from build123d import *
from build123d.topology import SkipClean

# Parameters (mm, degrees)
SKETCH_1_R          = 5.5
SKETCH_1_R_2        = 4.1
EXTRUDE_1_DEPTH     = 12.5
SKETCH_3_R          = 5.5
EXTRUDE_2_DEPTH     = 20
SKETCH_4_R          = 4.1
CUT_EXTRUDE_2_DEPTH = 22.5
SKETCH_5_R          = 4.1
CUT_EXTRUDE_3_DEPTH = 45


with BuildPart() as part:
    # 草图1 → 凸台-拉伸1 (new, symmetric)
    with BuildSketch(Plane(origin=(0, 0, 0), x_dir=(0, 0, -1), z_dir=(1, 0, 0))):
        Circle(SKETCH_1_R)
        Circle(SKETCH_1_R_2, mode=Mode.SUBTRACT)
    extrude(amount=EXTRUDE_1_DEPTH, both=True)

    # 草图3 → 凸台-拉伸2 (add)
    with BuildSketch(Plane(origin=(0, 0, 0), x_dir=(1, 0, 0), z_dir=(0, 1, 0))):
        with Locations(Location((0, 0, 0), (0, 0, 270))):
            Circle(SKETCH_3_R)
    extrude(amount=EXTRUDE_2_DEPTH)

    # 草图4 → 切除-拉伸2 (cut, symmetric)
    with SkipClean():  # the faces are left unmerged after this step: merging them gives an invalid solid
        with BuildSketch(Plane(origin=(0, 0, 0), x_dir=(0, 0, -1), z_dir=(1, 0, 0))):
            Circle(SKETCH_4_R)
        extrude(amount=CUT_EXTRUDE_2_DEPTH, both=True, mode=Mode.SUBTRACT)

    # 草图5 → 切除-拉伸3 (cut)
    with BuildSketch(Plane(origin=(0, 0, 0), x_dir=(1, 0, 0), z_dir=(0, 1, 0))):
        with Locations(Location((0, 0, 0), (0, 0, 270))):
            Circle(SKETCH_5_R)
    extrude(amount=CUT_EXTRUDE_3_DEPTH, mode=Mode.SUBTRACT)


solid = part.part
Can you work these out from the model? Positions are in its coordinate system, mm. A direction names the side the tool comes from. Give positions to 0.01 mm unless a question says otherwise; leave off trailing zeros. Order: outer loops, then holes, each group sorted by start corner. A loop starts at its lowest first (then second) coordinate and runs counter-clockwise, first axis right, second up. Notation, with made-up numbers: M 40.5,76 L 66.5,76 A11 cw 66.5,82 Z; hole C 9,35.5 d2. An arc over 180 degrees is marked long. Use one line per item in the form item = value.
Item 1: If we section it at A-A, the plane z = 0: Write out the boundary of the cut face in (x, y).
Values follow:
outline = M -12.5,-5.5 L 12.5,-5.5 L 12.5,-4.1 L -12.5,-4.1 Z; M -12.5,4.1 L -4.1,4.1 L -4.1,20 L -5.5,20 L -5.5,5.5 L -12.5,5.5 Z; M 4.1,4.1 L 12.5,4.1 L 12.5,5.5 L 5.5,5.5 L 5.5,20 L 4.1,20 Z
Item 2: If we section it at B-B, the plane x = 0: Write out the boundary of the cut face in (y, z).
Values follow:
outline = M 0,-5.5 L 20,-5.5 L 20,-4.1 L 0,-4.1 A4.1 cw 0,4.1 L 20,4.1 L 20,5.5 L 0,5.5 A5.5 ccw Z
Item 3: For faces 4 (the flat face through (-4, 20, -2)), 5 (the cylindrical face through (-5.37, 12.08, -1.19)), which set-ups out of +Z, -Z, +X, -X, +Y, -Y let a thin tool reach every point of the face, with its end or its side?
Values follow:
face_4 = +Z, -Z, +X, -X, +Y
face_5 = +Y
Item 4: If we section it at D-D, the plane x = 9.5: Write out the boundary of the cut face in (y, z).
Values follow:
outline = C 0,0 d11; hole C 0,0 d8.2
Item 5: Will these pins go through, and if not, where does the flat tip stop? pin 1 Ø5 at (y, z) = (-0.5, 3) entering from +X; pin 2 Ø1.5 at (x, y) = (5.5, 8) entering from +Z; pin 3 Ø1.5 at (x, z) = (-2.5, 2) entering from +Y; pin 4 Ø6 at (y, z) = (17, 0) entering from +X.
Values follow:
pin_1 = 12.5
pin_2 = 2.77
pin_3 = -3.04
pin_4 = 5.5
Item 6: If we section it at C-C, the plane y = -2: Write out the boundary of the cut face in (x, z), and give its area (3 significant figures).
Values follow:
outline = M -12.5,-5.12 L 12.5,-5.12 L 12.5,-3.58 L -12.5,-3.58 Z; M -12.5,3.58 L 12.5,3.58 L 12.5,5.12 L -12.5,5.12 Z
area = 77.2 mm^2
Item 7: If I drill on line 1 along Z through (x, y) = (3.25, 0); line 2 along X through (y, z) = (3.75, 3.25), over which ranges is the centre line in solid material (lowest first)? Write a range as [from, to].
Values follow:
line_1 = [-5.5, -4.1], [4.1, 5.5]
line_2 = [-12.5, -2.5], [2.5, 12.5]
Item 8: Thinking about a two-plate mould opening in Z: for faces 1 (the cylindrical face through (0.2, -4.9, -2.5)), 2 (the flat face through (-12.5, -4, 2)), 3 (the cylindrical face through (0.18, 12.082, -4.096)), which applies, pulls with the +Z half, pulls with the -Z half, needs draft (parallel to the pull), parting line crosses it, or undercut?
Values follow:
face_1 = parting line crosses it
face_2 = needs draft
face_3 = undercut
